```python
from build123d import *

# Parameters (mm, degrees)
CROQUIS1_R                 = 6
SALIENTE_EXTRUIR1_DEPTH    = 2.15
CROQUIS4_R                 = 4.65
SALIENTE_EXTRUIR3_DEPTH    = 7.2
CORTAR_EXTRUIR1_DEPTH      = 7.2
CORTAR_EXTRUIR1_DEPTH_BACK = 12.128342
CROQUIS2_R                 = 2.85
SALIENTE_EXTRUIR2_START    = -10
SALIENTE_EXTRUIR2_DEPTH    = 10
CHAFL_N1_SIZE              = 5.1
CHAFL_N1_SIZE2             = 0.975
SALIENTE_EXTRUIR4_DEPTH    = 9.2


with BuildPart() as part:
    # Croquis1 → Saliente-Extruir1 (new body)
    with BuildSketch(Plane(origin=(0, 0, 0), x_dir=(1, 0, 0), z_dir=(0, 1, 0))):
        with Locations(Location((0, 0, 0), (0, 0, 90))):
            Circle(CROQUIS1_R)
    extrude(amount=SALIENTE_EXTRUIR1_DEPTH)

    # Croquis4 → Saliente-Extruir3 (add)
    with BuildSketch(Plane(origin=(0, 2.15, 0), x_dir=(1, 0, 0), z_dir=(0, 1, 0))):
        with Locations(Location((0, 0, 0), (0, 0, 270))):
            Circle(CROQUIS4_R)
    extrude(amount=SALIENTE_EXTRUIR3_DEPTH)

    # Croquis2 → Cortar-Extruir1 (cut, two sides: drawn at the far end of the back side and taken through both)
    with BuildSketch(Plane(origin=(0, 2.15, 0), x_dir=(1, 0, 0), z_dir=(0, 1, 0)).offset(-CORTAR_EXTRUIR1_DEPTH_BACK)):
        with Locations(Location((0, 0, 0), (0, 0, 270))):
            Circle(CROQUIS2_R)
    extrude(amount=CORTAR_EXTRUIR1_DEPTH + CORTAR_EXTRUIR1_DEPTH_BACK, mode=Mode.SUBTRACT)

    # Croquis3 → Saliente-Extruir2 (add)
    with BuildSketch(Plane(origin=(0, 2.15, 0), x_dir=(1, 0, 0), z_dir=(0, 1, 0)).offset(SALIENTE_EXTRUIR2_START)):
        with BuildLine():
            Line((-5.279915, 2.85), (5.279915, 2.85))
            ThreePointArc((5.279915, 2.85), (0, 6), (-5.279915, 2.85))
        make_face()
    extrude(amount=SALIENTE_EXTRUIR2_DEPTH)

    # Chafl_n1
    chafl_n1_edges = [part.edges().sort_by_distance(p)[0] for p in [
        (0, 9.35, -4.65),
    ]]
    chafl_n1_side = [part.faces().sort_by_distance(p)[0] for p in [
        (0, 5.75, -4.65),
    ]]
    chamfer(chafl_n1_edges, length=CHAFL_N1_SIZE, length2=CHAFL_N1_SIZE2, reference=chafl_n1_side[0])

    # Croquis6 → Saliente-Extruir4 (add)
    with BuildSketch(Plane(origin=(0, 2.15, 0), x_dir=(1, 0, 0), z_dir=(0, 1, 0))):
        with BuildLine():
            Line((-4.524033, -1.075), (-2.639484, -1.075))
            ThreePointArc((-2.639484, -1.075), (-2.85, 0), (-2.639484, 1.075))
            Line((-2.639484, 1.075), (-4.524033, 1.075))
            ThreePointArc((-4.524033, 1.075), (-4.65, 0), (-4.524033, -1.075))
        make_face()
        with BuildLine():
            Line((1.075, -4.524033), (1.075, -2.639484))
            ThreePointArc((1.075, -2.639484), (0, -2.85), (-1.075, -2.639484))
            Line((-1.075, -2.639484), (-1.075, -4.524033))
            ThreePointArc((-1.075, -4.524033), (0, -4.65), (1.075, -4.524033))
        make_face()
        with BuildLine():
            Line((2.639484, 1.075), (4.524033, 1.075))
            ThreePointArc((4.524033, 1.075), (4.65, 0), (4.524033, -1.075))
            Line((4.524033, -1.075), (2.639484, -1.075))
            ThreePointArc((2.639484, -1.075), (2.85, 0), (2.639484, 1.075))
        make_face()
        with BuildLine():
            Line((-1.075, 2.639484), (-1.075, 4.524033))
            ThreePointArc((-1.075, 4.524033), (0, 4.65), (1.075, 4.524033))
            Line((1.075, 4.524033), (1.075, 2.639484))
            ThreePointArc((1.075, 2.639484), (0, 2.85), (-1.075, 2.639484))
        make_face()
    extrude(amount=SALIENTE_EXTRUIR4_DEPTH)


solid = part.part
```
CAD build for the part. Positions are in the model's coordinates, mm. A direction names the side the tool comes from. Round coordinates to 2 decimals unless told otherwise and drop trailing zeros. Order: outer loops, then holes, each group sorted by start corner. A loop starts at its lowest first (then second) coordinate and runs counter-clockwise, first axis right, second up.
Q1. Which spindle directions (+Z, -Z, +X, -X, +Y, -Y) get a long thin tool onto all of the face, cutting with end or side? Do faces 1 (the flat face through (4, 2.15, -3)), 2 (the flat face through (2.3, 9.35, 2.3)), 3 (the flat face through (-1.075, 9, 4)). Say none if no direction does.
Q2. Wall check: L1, parallel to Y at x = 3, z = 3.75; L2, parallel to X at y = 6.25, z = -1.75; L3, parallel to Z at x = -4.5, y = 4.5 (3 decimals). Give the ranges that are in metal, low to high.
Q3. Drop flat-ended pins along their axis: pin 1 (1.2 mm diameter, centred on x = 2, z = 3, fed in from +Y); pin 2 (2 mm diameter, centred on x = -3.5, y = -2.5, fed in from +Z); pin 3 (1.5 mm diameter, centred on y = 8.5, z = 3.5, fed in from -X); pin 4 (1 mm diameter, centred on x = 1, z = 0, fed in from -Y). Give the stop position or say it passes through.
Q4. Slice it at B-B (y = 3). Write the cut outline in (x, z), and give its area (3 significant figures).
Q5. Slice it at A-A (z = 0). Write the cut outline in (x, y), and give its area (3 significant figures).
Q6. Slice it at C-C (x = -5). Write the cut outline in (y, z), and give its area (3 significant figures).
Q7. Slice it at D-D (y = -2.5). Write the cut outline in (x, z), and give its area (3 significant figures).
Results below:
1. face 1: +Y
1. face 2: +Z, +X, +Y
1. face 3: +Z, -X, +Y
2. L1: y = 0 to 2.15
2. L2: x = -3.89 to -2.25, 2.25 to 3.89
2. L3: z = -1.075 to 1.075
3. pin 1: stops at y = 9.35
3. pin 2: stops at z = -2.85
3. pin 3: stops at x = -2.7
3. pin 4: passes through
4. outline: circle Ø9.3 at (0, 0); hole circle Ø5.7 at (0, 0)
4. area: 42.4 mm2
5. outline: (-6, 0) - (-2.85, 0) - (-2.85, 11.35) - (-4.65, 11.35) - (-4.65, 2.15) - (-6, 2.15) - close; (2.85, 0) - (6, 0) - (6, 2.15) - (4.65, 2.15) - (4.65, 11.35) - (2.85, 11.35) - close
5. area: 46.7 mm2
6. outline: (-7.85, -3.32) - (2.15, -3.32) - (2.15, 3.32) - (0, 3.32) - (0, -2.85) - (-7.85, -2.85) - close
6. area: 17.9 mm2
7. outline: (-5.28, -2.85) arc R6 ccw to (5.28, -2.85) - close
7. area: 23.7 mm2
